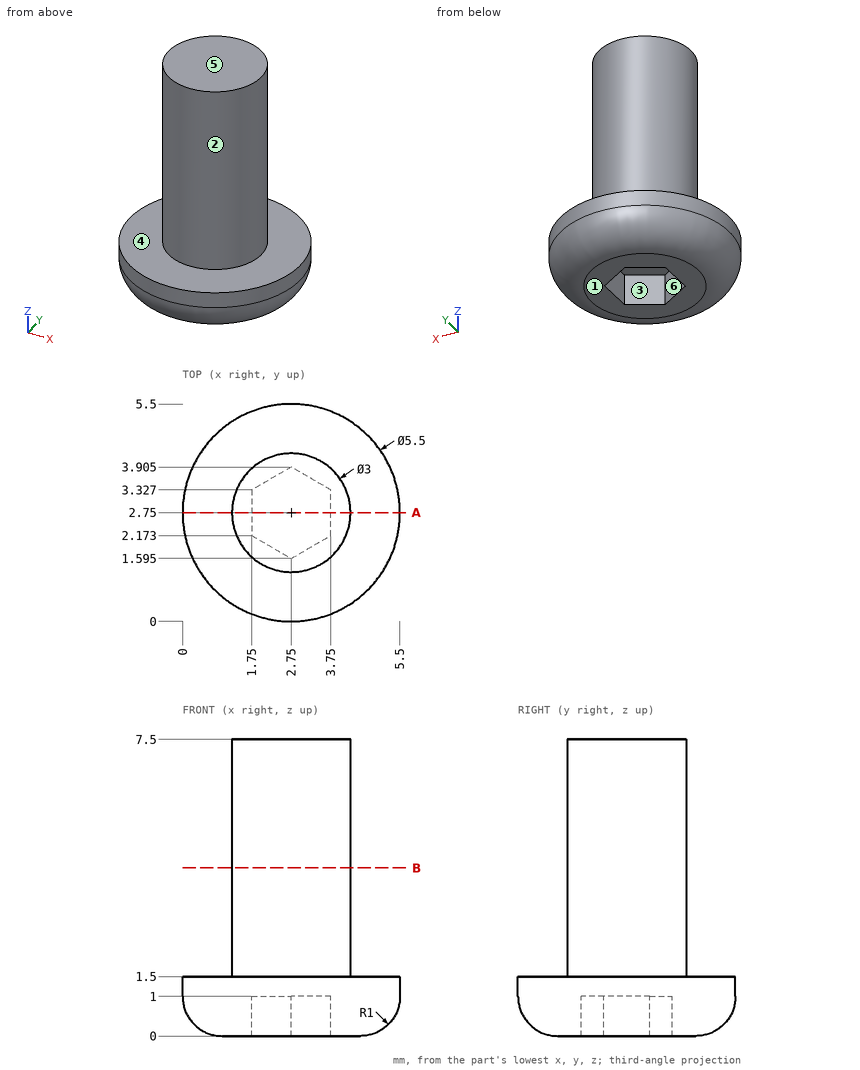
Design review of the part shown in the three views and the two pictorial views. Dimensions are in mm from the part's minimum x, y and z. A direction names the side the tool comes from. Give positions to 0.01 mm unless a question says otherwise; leave off trailing zeros. Loops run counter-clockwise (first coordinate to the right, second up) from the corner with the lowest first, then second, coordinate; pieces in that order, holes last. Notation, with made-up numbers: (-17, 31.5) - (42, 31.5) arc R29 ccw to (42, 51.5) - close; hole circle Ø7 at (-13, 86). An arc over 180 degrees is marked (long way). Answer as a JSON object with one key per item and string values.
Q1. Insertion check: pin 1 (0.8 mm diameter, centred on y = 3, z = 0.5, fed in from +X); pin 2 (1.5 mm diameter, centred on x = 1.5, z = 1.5, fed in from +Y); pin 3 (3 mm diameter, centred on x = 3.5, z = 6, fed in from -Y). Each pin has a flat end and moves straight along its axis. Give the tip position at first contact, or say it passes through.
Worked out:
{"pin 1": "stops at x = 5.49", "pin 2": "stops at y = 5.45", "pin 3": "stops at y = 1.25"}
Q2. To check wall thickness, follow line 1 along Y through (x, z) = (2.75, 5); line 2 along Z through (x, y) = (4.5, 3); line 3 along Z through (x, y) = (2.45, 2.8). State the ranges of each line that lie inside material, in increasing order.
Worked out:
{"line 1": "y = 1.25 to 4.25", "line 2": "z = 0 to 1.5", "line 3": "z = 1 to 7.5"}
Q3. Add section A-A on y = 2.75. State the section outline as (x, z) points.
Worked out:
{"outline": "(0, 1) arc R1 ccw to (1, 0) - (1.75, 0) - (1.75, 1) - (3.75, 1) - (3.75, 0) - (4.5, 0) arc R1 ccw to (5.5, 1) - (5.5, 1.5) - (4.25, 1.5) - (4.25, 7.5) - (1.25, 7.5) - (1.25, 1.5) - (0, 1.5) - close"}
Q4. For the marked faces 4, 5 and 6, list the 3-axis set-ups (+Z, -Z, +X, -X, +Y, -Y) from which the entire face can be reached by the end or side of a thin tool; tool diameter is ignored.
Worked out:
{"face 4": "+Z", "face 5": "+Z, +X, -X, +Y, -Y", "face 6": "-Z"}
Q5. Mouldability with a two-part tool opening along Y and no side actions: class the marked faces 1, 2 and 3 as +Y half, -Y half, draft (parallel to the pull), parting line (faces both ways), or undercut.
Worked out:
{"face 1": "draft", "face 2": "parting line", "face 3": "undercut"}
Q6. Add section B-B on z = 4.25. State the section outline as (x, y) points.
Worked out:
{"outline": "circle Ø3 at (2.75, 2.75)"}
